Verification items for the finished model (mm, model axes). A direction names the side the tool comes from. Round coordinates to 2 decimals unless told otherwise and drop trailing zeros. Write each loop counter-clockwise with the first axis right and the second up, starting at its lowest first coordinate (ties: lowest second). Pieces come first, ordered by that corner, then holes. Notation, with made-up numbers: (30, -35.5) - (70, -35.5) arc R34 cw to (70, -1.5) - close; hole circle Ø4 at (21, -38.5). An arc over 180 degrees is marked (long way). Write each question's results on one line, items separated by ' | '.
```python
from build123d import *

# Parameters (mm, degrees)
BOSS_EXTRUDE1_DEPTH = 30
CUT_EXTRUDE1_REACH  = 154.306
CUT_EXTRUDE2_DEPTH  = 19
SKETCH5_W           = 82.08
SKETCH5_H           = 54.14
CUT_EXTRUDE4_DEPTH  = 12.4
SKETCH4_R           = 1.25
CUT_EXTRUDE3_DEPTH  = 15
FILLET1_R           = 5
CUT_EXTRUDE5_DEPTH  = 5
BOSS_EXTRUDE2_DEPTH = 30
CUT_EXTRUDE6_REACH  = 160.176
SKETCH8_R           = 38
CUT_EXTRUDE7_REACH  = 179.588
SKETCH9_R           = 38
FILLET2_R           = 5
CUT_EXTRUDE8_REACH  = 106.763
SKETCH10_W          = 15
SKETCH10_H          = 4
SKETCH10_W_2        = 46
SKETCH10_H_2        = 6
CUT_EXTRUDE9_REACH  = 159.473
SKETCH11_R          = 1.25


with BuildPart() as part:
    # Sketch1 → Boss-Extrude1 (new body)
    with BuildSketch(Plane(origin=(0, 0, 0), x_dir=(1, 0, 0), z_dir=(0, 1, 0))):
        with BuildLine():
            Line((53, 80), (53, 129.147822281))
            ThreePointArc((53, 129.147822281), (0, 139.6), (-53, 129.147822281))
            Line((-53, 129.147822281), (-53, 80))
            Line((-53, 80), (-41, 68))
            Line((-41, 68), (41, 68))
            Line((41, 68), (53, 80))
        make_face()
    extrude(amount=BOSS_EXTRUDE1_DEPTH)

    # Sketch2 → Cut-Extrude1 (cut, up to next)
    with BuildSketch(Plane(origin=(0, 30, 0), x_dir=(1, 0, 0), z_dir=(0, 1, 0)), mode=Mode.PRIVATE) as cut_extrude1_sk1:
        Polygon((-49, 84), (49, 84), (49, 124), (27, 124), (27, 132), (-27, 132), (-27, 124), (-49, 124), align=None)
    cut_extrude1_tool1 = extrude(cut_extrude1_sk1.sketch, amount=-CUT_EXTRUDE1_REACH, mode=Mode.PRIVATE) & part.part
    add(cut_extrude1_tool1.solids().sort_by_distance((0, 30, -106.382353))[0], mode=Mode.SUBTRACT)

    # Sketch3 → Cut-Extrude2 (cut)
    with BuildSketch(Plane(origin=(0, 30, 0), x_dir=(1, 0, 0), z_dir=(0, 1, 0))):
        Polygon((-50.4, 125.280170906), (-50.4, 82.6), (50.4, 82.6), (50.4, 125.280170906), (28.070469991, 133.4), (-28.070469991, 133.4), align=None)
    extrude(amount=-CUT_EXTRUDE2_DEPTH, mode=Mode.SUBTRACT)

    # Sketch5 → Cut-Extrude4 (cut)
    with BuildSketch(Plane(origin=(0, 30, 0), x_dir=(1, 0, 0), z_dir=(0, 1, 0))):
        with Locations((-1.84, 98.58)):
            Rectangle(SKETCH5_W, SKETCH5_H)
    extrude(amount=-CUT_EXTRUDE4_DEPTH, mode=Mode.SUBTRACT)

    # Sketch4 → Cut-Extrude3 (cut)
    with BuildSketch(Plane(origin=(0, 17.6, 0), x_dir=(1, 0, 0), z_dir=(0, 1, 0))):
        with Locations(Location((26.18, 74.72, 0), (0, 0, 270))):
            Circle(SKETCH4_R)
        with Locations(Location((-27.53, 74.72, 0), (0, 0, 270))):
            Circle(SKETCH4_R)
    extrude(amount=-CUT_EXTRUDE3_DEPTH, mode=Mode.SUBTRACT)

    # Fillet1
    fillet1_edges = [part.edges().sort_by_distance(p)[0] for p in [
        (-42.88, 23.8, -71.51),
        (39.2, 23.8, -71.51),
    ]]
    fillet(fillet1_edges, radius=FILLET1_R)

    # Sketch6 → Cut-Extrude5 (cut)
    with BuildSketch(Plane(origin=(0, 30, 0), x_dir=(1, 0, 0), z_dir=(0, 1, 0))):
        with BuildLine():
            Line((50.4, 81.076955262), (50.4, 127.392464455))
            ThreePointArc((50.4, 127.392464455), (0, 137), (-50.4, 127.392464455))
            Line((-50.4, 127.392464455), (-50.4, 81.076955262))
            Line((-50.4, 81.076955262), (-39.923044738, 70.6))
            Line((-39.923044738, 70.6), (39.923044738, 70.6))
            Line((39.923044738, 70.6), (50.4, 81.076955262))
        make_face()
    extrude(amount=-CUT_EXTRUDE5_DEPTH, mode=Mode.SUBTRACT)

    # Sketch7 → Boss-Extrude2 (add)
    with BuildSketch(Plane.XZ):
        with BuildLine():
            Line((73.456296502, -118.711130498), (53, -98.254833996))
            Line((53, -98.254833996), (53, -129.147822281))
            ThreePointArc((53, -129.147822281), (63.443123072, -124.350834878), (73.456296502, -118.711130498))
        make_face()
    boss_extrude2 = extrude(amount=-BOSS_EXTRUDE2_DEPTH)

    # Cut-Extrude6: up to this plane
    cut_extrude6_end = Plane(origin=(53, 30, -80), z_dir=(-1, 0, 0))
    # Sketch8 → Cut-Extrude6 (cut, up to the surface)
    with BuildSketch(Plane(origin=(96.0837135, 0, -96.0837135), x_dir=(0, -1, 0), z_dir=(-0.7071067811865488, 0, 0.7071067811865464)), mode=Mode.PRIVATE) as cut_extrude6_sk1:
        with Locations((-26, 0)):
            Circle(SKETCH8_R)
    cut_extrude6_tool1 = split(extrude(cut_extrude6_sk1.sketch, amount=CUT_EXTRUDE6_REACH, mode=Mode.PRIVATE), bisect_by=cut_extrude6_end, keep=Keep.BOTH, mode=Mode.PRIVATE)
    add(cut_extrude6_tool1.solids().sort_by_distance((96.083714, 26, -96.083714))[0], mode=Mode.SUBTRACT)

    # Mirror1: Boss-Extrude2 across plane
    add(boss_extrude2.mirror(Plane(origin=(0, 0, 0), x_dir=(0, 0, 1), z_dir=(1, 0, 0))))

    # Cut-Extrude7: up to this plane
    cut_extrude7_end = Plane(origin=(-53, 30, -129.147822281), z_dir=(1, 0, 0))
    # Sketch9 → Cut-Extrude7 (cut, up to the surface)
    with BuildSketch(Plane(origin=(-96.0837135, 0, -96.0837135), x_dir=(0, -1, 0), z_dir=(0.7071067811865488, 0, 0.7071067811865464)), mode=Mode.PRIVATE) as cut_extrude7_sk1:
        with Locations((-26, 0)):
            Circle(SKETCH9_R)
    cut_extrude7_tool1 = split(extrude(cut_extrude7_sk1.sketch, amount=CUT_EXTRUDE7_REACH, mode=Mode.PRIVATE), bisect_by=cut_extrude7_end, keep=Keep.BOTH, mode=Mode.PRIVATE)
    add(cut_extrude7_tool1.solids().sort_by_distance((-96.083714, 26, -96.083714))[0], mode=Mode.SUBTRACT)

    # Fillet2
    fillet2_edges = [part.edges().sort_by_distance(p)[0] for p in [
        (68.992680179, 17.464833723, -121.359672387),
        (73.456296502, 2.753049234, -118.711130498),
        (-73.456296502, 2.753049234, -118.711130498),
        (-68.992679253, 17.464838179, -121.359672914),
    ]]
    fillet(fillet2_edges, radius=FILLET2_R - 0.0001)  # a hair under: the kernel refuses the full size

    # Sketch10 → Cut-Extrude8 (cut, up to next)
    with BuildSketch(Plane.XY.offset(-68), mode=Mode.PRIVATE) as cut_extrude8_sk1:
        with Locations((-40.5, 14)):
            Rectangle(SKETCH10_W, SKETCH10_H)
    cut_extrude8_tool1 = extrude(cut_extrude8_sk1.sketch, amount=-CUT_EXTRUDE8_REACH, mode=Mode.PRIVATE) & part.part
    # Sketch10 → Cut-Extrude8 (cut, up to next)
    with BuildSketch(Plane.XY.offset(-68), mode=Mode.PRIVATE) as cut_extrude8_sk2:
        with Locations((0, 15)):
            Rectangle(SKETCH10_W_2, SKETCH10_H_2)
    cut_extrude8_tool2 = extrude(cut_extrude8_sk2.sketch, amount=-CUT_EXTRUDE8_REACH, mode=Mode.PRIVATE) & part.part
    # Sketch10 → Cut-Extrude8 (cut, up to next)
    with BuildSketch(Plane.XY.offset(-68), mode=Mode.PRIVATE) as cut_extrude8_sk3:
        with Locations((40.5, 14)):
            Rectangle(SKETCH10_W, SKETCH10_H)
    cut_extrude8_tool3 = extrude(cut_extrude8_sk3.sketch, amount=-CUT_EXTRUDE8_REACH, mode=Mode.PRIVATE) & part.part
    add(cut_extrude8_tool1.solids().sort_by_distance((-40.5, 14, -68))[0], mode=Mode.SUBTRACT)
    add(cut_extrude8_tool2.solids().sort_by_distance((0, 15, -68))[0], mode=Mode.SUBTRACT)
    add(cut_extrude8_tool3.solids().sort_by_distance((40.5, 14, -68))[0], mode=Mode.SUBTRACT)

    # Sketch11 → Cut-Extrude9 (cut, up to next)
    with BuildSketch(Plane(origin=(0, 11, 0), x_dir=(1, 0, 0), z_dir=(0, 1, 0)), mode=Mode.PRIVATE) as cut_extrude9_sk1:
        with Locations(Location((-30, 128, 0), (0, 0, 270))):
            Circle(SKETCH11_R)
    cut_extrude9_tool1 = extrude(cut_extrude9_sk1.sketch, amount=-CUT_EXTRUDE9_REACH, mode=Mode.PRIVATE) & part.part
    # Sketch11 → Cut-Extrude9 (cut, up to next)
    with BuildSketch(Plane(origin=(0, 11, 0), x_dir=(1, 0, 0), z_dir=(0, 1, 0)), mode=Mode.PRIVATE) as cut_extrude9_sk2:
        with Locations(Location((30, 128, 0), (0, 0, 270))):
            Circle(SKETCH11_R)
    cut_extrude9_tool2 = extrude(cut_extrude9_sk2.sketch, amount=-CUT_EXTRUDE9_REACH, mode=Mode.PRIVATE) & part.part
    add(cut_extrude9_tool1.solids().sort_by_distance((-30, 11, -128))[0], mode=Mode.SUBTRACT)
    add(cut_extrude9_tool2.solids().sort_by_distance((30, 11, -128))[0], mode=Mode.SUBTRACT)


solid = part.part
```
(1) Go/stop test with flat-tipped pins: pin 1 Ø7 at (x, y) = (17.5, 15.5) entering from -Z; pin 2 Ø7.5 at (x, z) = (43.5, -76) entering from +Y; pin 3 Ø9.5 at (y, z) = (22, -110) entering from -X; pin 4 Ø4.5 at (x, z) = (0, -75.5) entering from +Y. Record where each tip stops, or that it passes through.
Answer:
pin 1: z = -138.9 | pin 2: y = 30 | pin 3: x = -61.37 | pin 4: y = 12
(2) Thickness scan on L1, parallel to X at y = 12.5, z = -74.72; L2, parallel to X at y = 28.5, z = -91; L3, parallel to X at y = 8, z = -74. Record the ranges inside material, lowest first.
Answer:
L1: -33 to -28.78, -26.28 to -23, 23 to 24.93, 27.43 to 33 | L2: -53 to -50.4, 50.4 to 53 | L3: -47 to -28.55, -26.51 to 25.16, 27.2 to 47
(3) Set-up check for faces 5 (the cylindrical face through (37.7, 21.25, -72.94)), 6 (the flat face through (27, 6, -128)), 7 (the flat face through (40, 16, -75)): record each of +Z, -Z, +X, -X, +Y, -Y from which the full face is reachable in a straight line by a thin tool's end or side.
Answer:
face 5: +Y | face 6: +Y, -Y | face 7: +Z
(4) Section check A-A (z = -92). Record the cut outline in (x, y), plus the area to 3 significant figures.
Answer:
outline: (-53, 0) - (-49, 0) - (-49, 11) - (-50.4, 11) - (-50.4, 30) - (-53, 30) - close; (49, 0) - (53, 0) - (53, 30) - (50.4, 30) - (50.4, 11) - (49, 11) - close | area: 187 mm2
(5) Section check B-B (x = 3.5). Record the cut outline in (y, z).
Answer:
outline: (0, -139.56) - (30, -139.56) - (30, -136.96) - (25, -136.96) - (25, -133.4) - (11, -133.4) - (11, -132) - (0, -132) - close; (0, -84) - (11, -84) - (11, -82.6) - (12, -82.6) - (12, -68) - (0, -68) - close; (18, -71.51) - (25, -71.51) - (25, -70.6) - (30, -70.6) - (30, -68) - (18, -68) - close
(6) Mould release check, pull along Y, two halves, no side actions. Record for faces 1 (the flat face through (0, 0, -82)), 2 (the flat face through (-50.4, 21, -105)), 3 (the flat face through (0, 25, -134)), 4 (the flat face through (-23, 15, -75)): released by +Y, released by -Y, zero draft, split by the parting line, or undercut.
Answer:
face 1: released by -Y | face 2: zero draft | face 3: released by +Y | face 4: undercut
